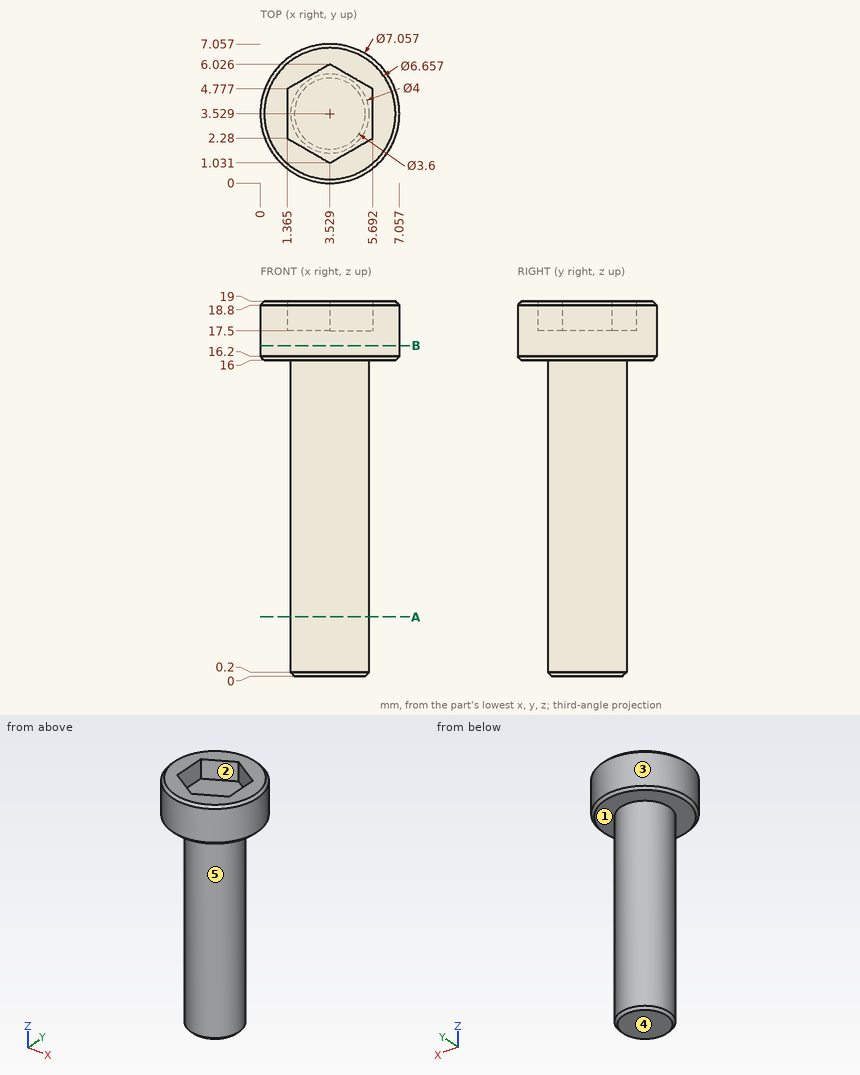
Design review of the part shown in the three views and the two pictorial views. Dimensions are in mm from the part's minimum x, y and z. A direction names the side the tool comes from. Give positions to 0.01 mm unless a question says otherwise; leave off trailing zeros. Write each loop counter-clockwise with the first axis right and the second up, starting at its lowest first coordinate (ties: lowest second). Pieces come first, ordered by that corner, then holes. Notation, with made-up numbers: M 39,-14.75 L 70,-14.75 A24 ccw 70,23.25 Z; hole C 85,28.5 d9. An arc over 180 degrees is marked long. One line per item, written item: value.
1) For line 1 (Z direction, x = 1, y = 5.5); line 2 (Y direction, x = 3.5, z = 11); line 3 (Z direction, x = 4.75, y = 2.5), list the stretches that pass through material, from the lowest coordinate up. Write a range as from..to.
Results are:
line 1: z = 16..19
line 2: y = 1.53..5.53
line 3: z = 0..17.5
2) Take a section at A-A, the plane z = 3. Write out the cut boundary in (x, y).
Results are:
outline: C 3.53,3.53 d4
3) The part is to be moulded in two halves that separate along Y. For the marked faces 1, 2 and 3, say which applies: +Y half, -Y half, draft (parallel to the pull), parting line (faces both ways), or undercut.
Results are:
face 1: draft
face 2: undercut
face 3: parting line
4) Take a section at B-B, the plane z = 16.75. Write out the cut boundary in (x, y).
Results are:
outline: C 3.53,3.53 d7.06
5) For the marked faces 4 and 5, list the 3-axis set-ups (+Z, -Z, +X, -X, +Y, -Y) from which the entire face can be reached by the end or side of a thin tool; tool diameter is ignored.
Results are:
face 4: -Z, +X, -X, +Y, -Y
face 5: -Z
6) For P1, Ø4, axis at y = 6, z = 5.5, coming from the +X side; P2, Ø1.5, axis at x = 5.5, z = 4, coming from the +Y side; P3, Ø1.5, axis at x = 5, z = 9, coming from the +Y side, all flat-tipped, find the tip position at first contact; note any pin that passes through.
Results are:
P1: stops at x = 5.47
P2: stops at y = 5.11
P3: stops at y = 5.39
